Source: CAD feature listing. Evaluate the final solid. Frame: model axes, mm. Face numbers are marked on the shaded views. A direction names the side the tool comes from. Coordinates: 2 decimals unless noted, no trailing zeros. Loops run counter-clockwise (first coordinate to the right, second up) from the corner with the lowest first, then second, coordinate; pieces in that order, holes last. Notation, with made-up numbers: (73.5, 82.25) - (98.5, 82.25) arc R10 ccw to (98.5, 90.25) - close; hole circle Ø8 at (8, 51.5). An arc over 180 degrees is marked (long way). Use one line per item in the form item = value. Start each with the question number.
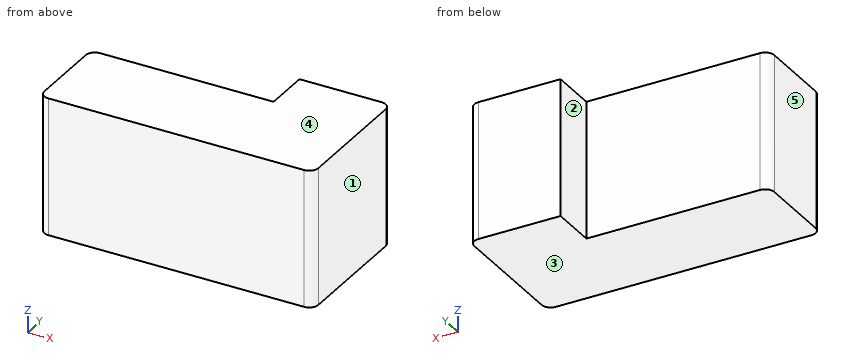
from build123d import *

# Parameters (mm, degrees)
F1_DEPTH = 50.8
F2_R     = 5.08
F3_R     = 5.08
F4_DEPTH = 76.2
F5_R     = 5.08


with BuildPart() as f1:
    # F0 (on Top) → F1 (new body)
    with BuildSketch(Plane.XY):
        Polygon((0, 50.8), (0, 0), (152.4, 0), (152.4, 76.2), (101.6, 76.2), (101.6, 50.8), align=None)
    extrude(amount=F1_DEPTH)

    # F2
    f2_edges = [f1.edges().sort_by_distance(p)[0] for p in [
        (0, 0, 25.4),
        (0, 50.8, 25.4),
        (152.4, 0, 25.4),
    ]]
    fillet(f2_edges, radius=F2_R)

    # F3
    f3_edges = [f1.edges().sort_by_distance(p)[0] for p in [
        (152.4, 76.2, 25.4),
    ]]
    fillet(f3_edges, radius=F3_R)

    # F0 (on Top) → F4 (join)
    with BuildSketch(Plane.XY):
        Polygon((0, 50.8), (0, 0), (152.4, 0), (152.4, 76.2), (101.6, 76.2), (101.6, 50.8), align=None)
    extrude(amount=F4_DEPTH)

    # F5
    f5_edges = [f1.edges().sort_by_distance(p)[0] for p in [
        (152.4, 76.2, 38.1),
        (152.4, 0, 38.1),
        (0, 0, 38.1),
        (0, 50.8, 38.1),
    ]]
    fillet(f5_edges, radius=F5_R)


solid = f1.part
(1) Contact query for flat-ended pins moving along their axis: pin 1 (2 mm diameter, centred on y = 61, z = 59.5, fed in from -X); pin 2 (3 mm diameter, centred on x = 71, y = 35, fed in from -Z). Output: stop coordinate, or through.
(2) Mould query, pull axis Z, two halves, no side actions, for the marked faces 3, 4 and 5. Classes: +Z half, -Z half, draft (parallel to the pull), parting line (faces both ways), or undercut.
(3) Material intervals for line 1 (Y direction, x = 101, z = 11.5); line 2 (X direction, y = 5, z = 44); line 3 (X direction, y = 66.5, z = 44.5), sorted ascending.
(4) Cut plane A-A, the plane z = 37. Output: boundary loops of the cut face in (x, y).
(5) Access query for the marked faces 1 and 2. Directions: +Z, -Z, +X, -X, +Y, -Y. A direction counts if a zero-diameter tool reaches every point of the face in a straight line with its end or side. Return the directions, or none.
(6) Cut plane C-C, the plane x = 66. Output: boundary loops of the cut face in (y, z), plus the area to 3 significant figures.
(7) Cut plane B-B, the plane y = 68.5. Output: boundary loops of the cut face in (x, z), plus the area to 3 significant figures.
Recorded:
q1.pin_1 = 101.6
q1.pin_2 = 0
q2.face_3 = -Z half
q2.face_4 = +Z half
q2.face_5 = draft
q3.line_1 = 0 to 50.8
q3.line_2 = 0 to 152.4
q3.line_3 = 101.6 to 152.4
q4.outline = (0, 5.08) arc R5.08 ccw to (5.08, 0) - (147.32, 0) arc R5.08 ccw to (152.4, 5.08) - (152.4, 71.12) arc R5.08 ccw to (147.32, 76.2) - (101.6, 76.2) - (101.6, 50.8) - (5.08, 50.8) arc R5.08 ccw to (0, 45.72) - close
q5.face_1 = +Z, -Z, +X, +Y, -Y
q5.face_2 = +Z, -Z, -X, +Y
q6.outline = (0, 0) - (50.8, 0) - (50.8, 76.2) - (0, 76.2) - close
q6.area = 3,870 mm²
q7.outline = (101.6, 0) - (152.4, 0) - (152.4, 76.2) - (101.6, 76.2) - close
q7.area = 3,870 mm²
